Design review of the part built by this model. Coordinates are the model's own, in mm. A direction names the side the tool comes from. Give positions to 0.01 mm unless a question says otherwise; leave off trailing zeros. Order: outer loops, then holes, each group sorted by start corner. A loop starts at its lowest first (then second) coordinate and runs counter-clockwise, first axis right, second up. Notation, with made-up numbers: (43.5, -0.75) -> (47.5, -0.75) arc R27 ccw to (47.5, 21.25) -> close; hole circle Ø2 at (-19.75, 47). An arc over 180 degrees is marked (long way). Use a Markdown table: item, result. Add a question column.
```python
from build123d import *

# Parameters (mm, degrees)
SKETCH1_R           = 7.5
SKETCH1_R_2         = 5
BOSS_EXTRUDE1_DEPTH = 41
SKETCH2_W           = 80
SKETCH2_H           = 20
BOSS_EXTRUDE2_DEPTH = 150
SKETCH3_R           = 5
CUT_EXTRUDE1_DEPTH  = 150
CUT_EXTRUDE2_DEPTH  = 150
CUT_EXTRUDE3_DEPTH  = 6
FILLET1_R           = 6


with BuildPart() as part:
    # Sketch1 → Boss-Extrude1 (new body)
    with BuildSketch(Plane.XY):
        Circle(SKETCH1_R)
        Circle(SKETCH1_R_2, mode=Mode.SUBTRACT)
    extrude(amount=BOSS_EXTRUDE1_DEPTH)

    # Sketch2 → Boss-Extrude2 (add)
    with BuildSketch(Plane(origin=(0, 0, 0), x_dir=(1, 0, 0), z_dir=(0, 1, 0))):
        with Locations((0, -20.5)):
            Rectangle(SKETCH2_W, SKETCH2_H)
    extrude(amount=BOSS_EXTRUDE2_DEPTH)

    # Sketch3 → Cut-Extrude1 (cut)
    with BuildSketch(Plane(origin=(0, 0, 0), x_dir=(-1, 0, 0), z_dir=(0, 0, -1))):
        with Locations(Location((0, 0, 0), (0, 0, 180))):
            Circle(SKETCH3_R)
    extrude(amount=-CUT_EXTRUDE1_DEPTH, mode=Mode.SUBTRACT)

    # Sketch4 → Cut-Extrude2 (cut)
    with BuildSketch(Plane(origin=(0, 0, 10.5), x_dir=(-1, 0, 0), z_dir=(0, 0, -1))):
        Polygon((7.5, 0), (40, 150), (40, 0), align=None)
    cut_extrude2 = extrude(amount=-CUT_EXTRUDE2_DEPTH, mode=Mode.SUBTRACT)

    # Mirror1: Cut-Extrude2 across plane
    add(cut_extrude2.mirror(Plane(origin=(0, 0, 0), x_dir=(0, 0, 1), z_dir=(1, 0, 0))), mode=Mode.SUBTRACT)

    # Sketch5 → Cut-Extrude3 (cut)
    with BuildSketch(Plane.XY.offset(30.5)):
        Polygon((-28, 144.230769231), (0, 15), (28, 144.230769231), align=None)
    cut_extrude3 = extrude(amount=-CUT_EXTRUDE3_DEPTH, mode=Mode.SUBTRACT)

    # Mirror2: Cut-Extrude3 across plane
    add(cut_extrude3.mirror(Plane.XY.offset(20)), mode=Mode.SUBTRACT)

    # Fillet1
    # the kernel refuses this fillet: 6 mm, written as the material it adds along each edge
    with BuildSketch(Plane(origin=(-3.176300205, 0.3401529, 24.5), x_dir=(0, 0, 1), z_dir=(0.21175334700580606, 0.9773231400267973, 0))) as fillet1_piece_1_section:
        with BuildLine():
            CenterArc((FILLET1_R, -FILLET1_R), FILLET1_R, 90, 90)
            Line((0, -FILLET1_R), (0, 0))
            Line((0, 0), (FILLET1_R, 0))
        make_face()
    fillet1_piece_1 = extrude(amount=162.229314889, mode=Mode.PRIVATE)
    fillet1_piece_1 = split(fillet1_piece_1, bisect_by=Plane(origin=(-13.111456884, 75.514416388, 25.854154081), z_dir=(0.9773231400267973, 0.21175334700580611, 0)), keep=Keep.TOP, mode=Mode.PRIVATE)
    fillet1_piece_1 = split(fillet1_piece_1, bisect_by=Plane(origin=(12.989714393, 144.230769231, 25.854154081), z_dir=(0, -1, 0)), keep=Keep.TOP, mode=Mode.PRIVATE)
    add(fillet1_piece_1)
    with BuildSketch(Plane(origin=(-31.176300205, 158.890616331, 24.5), x_dir=(0, 0, 1), z_dir=(0.21175334700580611, -0.9773231400267973, 0))) as fillet1_piece_2_section:
        with BuildLine():
            CenterArc((FILLET1_R, -FILLET1_R), FILLET1_R, 90, 90)
            Line((0, -FILLET1_R), (0, 0))
            Line((0, 0), (FILLET1_R, 0))
        make_face()
    fillet1_piece_2 = extrude(amount=162.229314889, mode=Mode.PRIVATE)
    fillet1_piece_2 = split(fillet1_piece_2, bisect_by=Plane(origin=(13.111456884, 75.514416388, 25.854154081), z_dir=(-0.9773231400267973, 0.21175334700580606, 0)), keep=Keep.TOP, mode=Mode.PRIVATE)
    fillet1_piece_2 = split(fillet1_piece_2, bisect_by=Plane(origin=(-12.989714393, 144.230769231, 25.854154081), z_dir=(0, -1, 0)), keep=Keep.TOP, mode=Mode.PRIVATE)
    add(fillet1_piece_2)
    with BuildSketch(Plane(origin=(43, 144.230769231, 24.5), x_dir=(0, 0, 1), z_dir=(-1, 0, 0))) as fillet1_piece_3_section:
        with BuildLine():
            CenterArc((FILLET1_R, -FILLET1_R), FILLET1_R, 90, 90)
            Line((0, -FILLET1_R), (0, 0))
            Line((0, 0), (FILLET1_R, 0))
        make_face()
    fillet1_piece_3 = extrude(amount=86, mode=Mode.PRIVATE)
    fillet1_piece_3 = split(fillet1_piece_3, bisect_by=Plane(origin=(-26.469184818, 137.165468391, 25.846029793), z_dir=(0.9773231400267973, 0.21175334700580611, 0)), keep=Keep.TOP, mode=Mode.PRIVATE)
    fillet1_piece_3 = split(fillet1_piece_3, bisect_by=Plane(origin=(26.469184818, 137.165468391, 25.846029793), z_dir=(-0.9773231400267973, 0.21175334700580606, 0)), keep=Keep.TOP, mode=Mode.PRIVATE)
    add(fillet1_piece_3)
    with BuildSketch(Plane(origin=(-3.131874238, 0.545195824, 15.5), x_dir=(0, 0, -1), z_dir=(0.21175334700580606, 0.9773231400267973, 0))) as fillet1_piece_4_section:
        with BuildLine():
            CenterArc((6, 5.916079783), FILLET1_R, 180, 80.405931773)
            Line((0, 5.916079783), (0, 0))
            Line((0, 0), (5, 0))
        make_face()
    fillet1_piece_4 = extrude(amount=161.809713804, mode=Mode.PRIVATE)
    fillet1_piece_4 = split(fillet1_piece_4, bisect_by=Plane(origin=(12.010804887, 144.230769231, 14.091740846), z_dir=(0, -1, 0)), keep=Keep.TOP, mode=Mode.PRIVATE)
    fillet1_piece_4 = split(fillet1_piece_4, bisect_by=Plane(origin=(-12.92288351, 74.644077737, 14.091740846), z_dir=(0.9773231400267973, 0.21175334700580611, 0)), keep=Keep.TOP, mode=Mode.PRIVATE)
    add(fillet1_piece_4)
    with BuildSketch(Plane(origin=(-31.131874238, 158.685573406, 15.5), x_dir=(0, 0, -1), z_dir=(0.21175334700580611, -0.9773231400267973, 0))) as fillet1_piece_5_section:
        with BuildLine():
            CenterArc((6, 5.916079783), FILLET1_R, 180, 80.405931773)
            Line((0, 5.916079783), (0, 0))
            Line((0, 0), (5, 0))
        make_face()
    fillet1_piece_5 = extrude(amount=161.809713804, mode=Mode.PRIVATE)
    fillet1_piece_5 = split(fillet1_piece_5, bisect_by=Plane(origin=(-12.010804887, 144.230769231, 14.091740846), z_dir=(0, -1, 0)), keep=Keep.TOP, mode=Mode.PRIVATE)
    fillet1_piece_5 = split(fillet1_piece_5, bisect_by=Plane(origin=(12.92288351, 74.644077737, 14.091740846), z_dir=(-0.9773231400267973, 0.21175334700580606, 0)), keep=Keep.TOP, mode=Mode.PRIVATE)
    add(fillet1_piece_5)
    with BuildSketch(Plane(origin=(42.790199458, 144.230769231, 15.5), x_dir=(0, 0, -1), z_dir=(-1, 0, 0))) as fillet1_piece_6_section:
        with BuildLine():
            CenterArc((6, 5.916079783), FILLET1_R, 180, 80.405931773)
            Line((0, 5.916079783), (0, 0))
            Line((0, 0), (5, 0))
        make_face()
    fillet1_piece_6 = extrude(amount=85.580398916, mode=Mode.PRIVATE)
    fillet1_piece_6 = split(fillet1_piece_6, bisect_by=Plane(origin=(26.323275838, 136.492042329, 14.091740846), z_dir=(-0.9773231400267973, 0.21175334700580606, 0)), keep=Keep.TOP, mode=Mode.PRIVATE)
    fillet1_piece_6 = split(fillet1_piece_6, bisect_by=Plane(origin=(-26.323275838, 136.492042329, 14.091740846), z_dir=(0.9773231400267973, 0.21175334700580611, 0)), keep=Keep.TOP, mode=Mode.PRIVATE)
    add(fillet1_piece_6)


solid = part.part
```
1) Add section A-A (z = 5). Give the boundary of the cut face in (x, y), then the cut area to 3 significant figures.
2) Insertion check: pin 1 (12 mm diameter, centred on y = 54, z = 21, fed in from +X); pin 2 (12.5 mm diameter, centred on x = 1, y = 72.5, fed in from +Z); pin 3 (5 mm diameter, centred on x = 18.5, y = 96.5, fed in from -Z). Each pin has a flat end and moves straight along its axis. Give the tip position at first contact, or say it passes through.
3) Machinability: for faces 1 (the flat face through (0, 102, 15.5)), 2 (the cylindrical face through (-1.63, -7.32, 20.21)), 3 (the flat face through (-1, 150, 20)), 4 (the cylindrical face through (0.392, 142.52, 26.304)), which of the approach directions +Z, -Z, +X, -X, +Y, -Y give a long, thin tool a straight path to every point of the face, cutting with its end or side? Answer none if there is none.
4) Add section B-B (z = 27). Give the boundary of the cut face in (x, y), then the cut area to 3 significant figures.
5) Add section C-C (y = 11.5). Give the boundary of the cut face in (x, z).
6) The part is to be moulded in two halves that separate along Y. For faces 5 (the flat face through (-23.523, 73.95, 20.36)), 6 (the flat face through (2, -5, 0)), 7 (the cylindrical face through (-1.08, -4.88, 20.21)), say which applies: +Y half, -Y half, draft (parallel to the pull), parting line (faces both ways), or undercut.
7) For L1, parallel to Y at x = 0, z = 20; L2, parallel to Y at x = 3, z = 16; L3, parallel to Z at x = 26.5, y = 99.5, list the stretches that pass through material, from the lowest coordinate up. Write a range as [from, to].
Worked answers:
| question | item | result |
|---|---|---|
| 1 | outline | circle Ø15 at (0, 0); hole circle Ø10 at (0, 0) |
| 1 | area | 98.2 mm^2 |
| 2 | pin 1 | x = 20.5 |
| 2 | pin 2 | z = 24.59 |
| 2 | pin 3 | z = 10.5 |
| 3 | face 1 | -Z |
| 3 | face 2 | none |
| 3 | face 3 | +Z, -Z, +X, -X, +Y |
| 3 | face 4 | +Z |
| 4 | outline | (-40, 150) -> (-7.5, 0) arc R7.5 ccw to (7.5, 0) -> (40, 150) -> close; hole (-26.6, 143.1) -> (0, 20.32) -> (26.6, 143.1) -> close; hole circle Ø10 at (0, 0) |
| 4 | area | 3,870 mm^2 |
| 5 | outline | (-9.99, 10.5) -> (9.99, 10.5) -> (9.99, 30.5) -> (-9.99, 30.5) -> close |
| 6 | face 5 | -Y half |
| 6 | face 6 | draft |
| 6 | face 7 | undercut |
| 7 | L1 | [-7.5, -5], [5, 150] |
| 7 | L2 | [-6.87, -4], [4, 150] |
| 7 | L3 | [10.5, 30.5] |
